from build123d import *

# Parameters (mm, degrees)
SKETCH_1_R      = 20
SKETCH_1_R_2    = 15.1
EXTRUDE_1_DEPTH = 10
FILLET_1_R      = 2
SKETCH_2_W      = 3
SKETCH_2_H      = 5
SKETCH_2_W_2    = 5
SKETCH_2_H_2    = 3
EXTRUDE_2_DEPTH = 6


with BuildPart() as part:
    # Эскиз1 → Бобышка-Вытянуть1 (new body)
    with BuildSketch(Plane(origin=(0, 0, 0), x_dir=(1, 0, 0), z_dir=(0, 1, 0))):
        Circle(SKETCH_1_R)
        Circle(SKETCH_1_R_2, mode=Mode.SUBTRACT)
    extrude(amount=EXTRUDE_1_DEPTH)

    # Скругление1
    fillet_1_edges = [part.edges().sort_by_distance(p)[0] for p in [
        (-20, 0, 0),
        (-20, 10, 0),
    ]]
    fillet(fillet_1_edges, radius=FILLET_1_R)

    # Эскиз2 → Бобышка-Вытянуть2 (add)
    with BuildSketch(Plane(origin=(0, 10, 0), x_dir=(1, 0, 0), z_dir=(0, 1, 0))):
        with Locations((0, 15.1)):
            Rectangle(SKETCH_2_W, SKETCH_2_H)
        with Locations((-15.1, 0)):
            Rectangle(SKETCH_2_W_2, SKETCH_2_H_2)
        with Locations((15.1, 0)):
            Rectangle(SKETCH_2_W_2, SKETCH_2_H_2)
        with Locations((0, -15.1)):
            Rectangle(SKETCH_2_W, SKETCH_2_H)
    extrude(amount=-EXTRUDE_2_DEPTH)


solid = part.part
Can you work these out from the model? Positions are in its coordinate system, mm. A direction names the side the tool comes from. Give positions to 0.01 mm unless a question says otherwise; leave off trailing zeros. Loops run counter-clockwise (first coordinate to the right, second up) from the corner with the lowest first, then second, coordinate; pieces in that order, holes last. Notation, with made-up numbers: (-24.5, 88.5) -> (-4.5, 88.5) arc R20 ccw to (-4.5, 122.5) -> close; hole circle Ø6 at (71, 29.5). An arc over 180 degrees is marked (long way). Write item = value, one per line.
1) Suppose I cut it at B-B on x = 0. Write out the boundary of the cut face in (y, z).
Check result:
outline = (0, -18) arc R2 ccw to (2, -20) -> (8, -20) arc R2 ccw to (10, -18) -> (10, -12.6) -> (4, -12.6) -> (4, -15.1) -> (0, -15.1) -> close; (0, 15.1) -> (4, 15.1) -> (4, 12.6) -> (10, 12.6) -> (10, 18) arc R2 ccw to (8, 20) -> (2, 20) arc R2 ccw to (0, 18) -> close
2) Will these pins go through, and if not, where does the flat tip stop? pin 1 (0.9 mm diameter, centred on x = 0.5, y = 7.5, fed in from -Z); pin 2 (0.8 mm diameter, centred on x = 0, z = 14, fed in from -Y); pin 3 (1 mm diameter, centred on y = 6.5, z = 6, fed in from +X).
Check result:
pin_1 = -20
pin_2 = 4
pin_3 = 19.23
3) Suppose I cut it at A-A on z = 0. Write out the boundary of the cut face in (x, y).
Check result:
outline = (-20, 2) arc R2 ccw to (-18, 0) -> (-15.1, 0) -> (-15.1, 4) -> (-12.6, 4) -> (-12.6, 10) -> (-18, 10) arc R2 ccw to (-20, 8) -> close; (12.6, 4) -> (15.1, 4) -> (15.1, 0) -> (18, 0) arc R2 ccw to (20, 2) -> (20, 8) arc R2 ccw to (18, 10) -> (12.6, 10) -> close
4) Suppose I cut it at D-D on z = 14.5. Give the number of separate pieces and of enclosed holes in the cut face, then the cut area to 3 significant figures.
Check result:
separate_pieces = 3
enclosed_holes = 0
area = 204 mm2
5) I need wall thicknesses on L1, parallel to X at y = 7, z = -14; L2, parallel to X at y = 5.75, z = 0. Which ranges of each line are inside material? Lowest first, please. Write a range as from..to.
Check result:
L1 = -14.28..-5.66, -1.5..1.5, 5.66..14.28
L2 = -20..-12.6, 12.6..20
6) Thinking about a two-plate mould opening in X: for faces 4 (the cylindrical face through (-4.336, 4.958, 19.524)), 5 (the flat face through (0, 10, -13)), 6 (the flat face through (-14, 7, 1.5)), which applies, released by +X, released by -X, zero draft, split by the parting line, or undercut?
Check result:
face_4 = split by the parting line
face_5 = zero draft
face_6 = undercut
7) Suppose I cut it at C-C on y = 7. Write out the boundary of the cut face in (x, z), then the cut area to 3 significant figures.
Check result:
outline = circle Ø40 at (0, 0); hole (-15.03, -1.5) arc R15.1 ccw to (-1.5, -15.03) -> (-1.5, -12.6) -> (1.5, -12.6) -> (1.5, -15.03) arc R15.1 ccw to (15.03, -1.5) -> (12.6, -1.5) -> (12.6, 1.5) -> (15.03, 1.5) arc R15.1 ccw to (1.5, 15.03) -> (1.5, 12.6) -> (-1.5, 12.6) -> (-1.5, 15.03) arc R15.1 ccw to (-15.03, 1.5) -> (-12.6, 1.5) -> (-12.6, -1.5) -> close
area = 570 mm2
8) For faces 1 (the flat face through (-4, 0, -15)), 2 (the flat face through (0, 4, 14)), 3 (the flat face through (12.6, 7, 0)), which set-ups out of +Z, -Z, +X, -X, +Y, -Y let a thin tool reach every point of the face, with its end or its side?
Check result:
face_1 = +Z, -Z, +X, -X, -Y
face_2 = -Y
face_3 = +Y, -Y
